```python
from build123d import *

# Parameters (mm, degrees)
F1_DEPTH    = 6
F2_T1_DEPTH = 28.6290423826
F3_W        = 12.6199351555
F3_H        = 2
F3_W_2      = 15.3329153147
F4_DEPTH    = 6


# Not quite as in the source:
# - a fillet or chamfer that OpenCascade refuses, or shapes differently, is made with other operations: its cross-section is extruded or revolved along the edge and cut away or added


with BuildPart() as f1:
    # F0 (on Top) → F1 (new body)
    with BuildSketch(Plane.XY):
        Polygon((0, 7), (-7, 5), (0, 5), align=None)
        Polygon((0, 5), (-7, 5), (-7, 0), (0, 0), (11, 0), (18, 0), (18, 5), (11, 5), align=None)
        Polygon((0, 0), (-7, 0), (0, -2), align=None)
        Polygon((11, 7), (11, 5), (18, 5), align=None)
        Polygon((18, 0), (11, 0), (11, -2), align=None)
    extrude(amount=F1_DEPTH)

    # F2: fillet of radius 6 on 4 edges, made by hand

    # F2_s2 → F2_t1 (cut)
    with BuildSketch(Plane.XY.offset(-11.3145211913)):
        with BuildLine():
            ThreePointArc((-2.6483267674, 6.2433352093), (-5.7900918887, 4.0873646023), (-7, 0.4741915235))
            Line((-7, 0.4741915235), (-7, 5))
            Line((-7, 5), (-2.6483267674, 6.2433352093))
        make_face()
        with BuildLine():
            ThreePointArc((-7, 4.5258084765), (-5.7900918887, 0.9126353977), (-2.6483267674, -1.2433352093))
            Line((-2.6483267674, -1.2433352093), (-7, 0))
            Line((-7, 0), (-7, 4.5258084765))
        make_face()
        with BuildLine():
            ThreePointArc((18, 0.4741915235), (16.7900918887, 4.0873646023), (13.6483267674, 6.2433352093))
            Line((13.6483267674, 6.2433352093), (18, 5))
            Line((18, 5), (18, 0.4741915235))
        make_face()
        with BuildLine():
            ThreePointArc((13.6483267674, -1.2433352093), (16.7900918887, 0.9126353977), (18, 4.5258084765))
            Line((18, 4.5258084765), (18, 0))
            Line((18, 0), (13.6483267674, -1.2433352093))
        make_face()
    extrude(amount=F2_T1_DEPTH, mode=Mode.SUBTRACT)

    # F3 (on face) → F4 (cut)
    with BuildSketch(Plane.XY.offset(6)):
        with Locations((-2.9576308128, 2.5)):
            Rectangle(F3_W, F3_H)
        with Locations((15.3141208924, 2.5)):
            Rectangle(F3_W_2, F3_H)
    extrude(amount=-F4_DEPTH, mode=Mode.SUBTRACT)


solid = f1.part
```
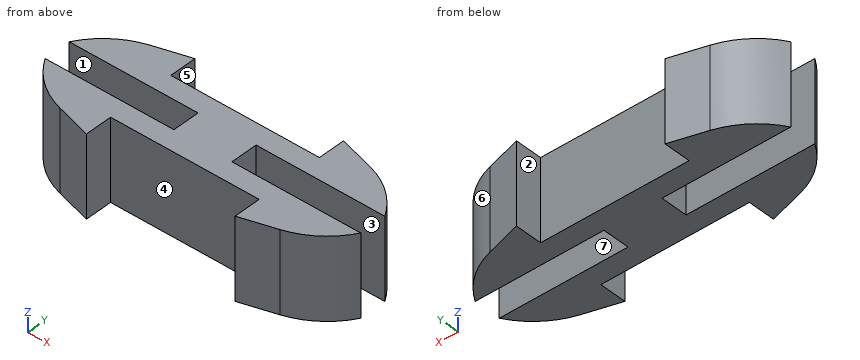
For this review, take the finished solid that the model builds, in its own axes (mm). Face numbers are marked on the shaded views. A direction names the side the tool comes from. Round coordinates to 2 decimals unless told otherwise and drop trailing zeros. Write each loop counter-clockwise with the first axis right and the second up, starting at its lowest first coordinate (ties: lowest second). Pieces come first, ordered by that corner, then holes. Notation, with made-up numbers: (89.25, 10.5) -> (105.25, 10.5) arc R15 cw to (105.25, 21.5) -> close; hole circle Ø3 at (-40, 56). An arc over 180 degrees is marked (long way). One line per question, with ' | ' between items. Start each with the question number.
(1) Mouldability with a two-part tool opening along X and no side actions: class the marked faces 4, 5, 6 and 7 as released by +X, released by -X, zero draft, split by the parting line, or undercut.
(2) Insertion check: P1, Ø1.6, axis at y = -1, z = 2.5, coming from the -X side; P2, Ø0.6, axis at y = 2.5, z = 3, coming from the -X side; P3, Ø2, axis at y = 6, z = 4.5, coming from the -X side. Each pin has a flat end and moves straight along its axis. Give the tip position at first contact, or say it passes through.
(3) Add section A-A, the plane x = 0.5. Write out the cut boundary in (y, z).
(4) Tool access review of the marked faces 1, 2 and 3: name each direction out of +Z, -Z, +X, -X, +Y, -Y from which nothing blocks a thin tool from reaching the whole face with its end or side.
(5) Add section C-C, the plane z = 3.25. Write out the cut boundary in (x, y), plus the area to 3 significant figures.
(6) Add section D-D, the plane y = 3.25. Write out the cut boundary in (x, z).
(7) For line 1 along Y through (x, z) = (3, 1.5); line 2 along Y through (x, z) = (-1.5, 2.5); line 3 along X through (y, z) = (2, 1), list the stretches that pass through material, from the lowest coordinate up. Write a range as from..to.
(8) Add section B-B, the plane y = 6.5. Write out the cut boundary in (x, z), plus the area to 3 significant figures.
Answer list:
1) face 4: undercut | face 5: undercut | face 6: released by +X | face 7: zero draft
2) P1: x = -4.7 | P2: x = 3.35 | P3: x = -4.94
3) outline: (0, 0) -> (1.5, 0) -> (1.5, 6) -> (0, 6) -> close; (3.5, 0) -> (5, 0) -> (5, 6) -> (3.5, 6) -> close
4) face 1: +Z, -Z, -X | face 2: +Z, -Z, +Y | face 3: +Z, -Z, +X
5) outline: (-6.18, 1.5) arc R6 ccw to (-2.65, -1.24) -> (0, -2) -> (0, 0) -> (11, 0) -> (11, -2) -> (13.65, -1.24) arc R6 ccw to (17.18, 1.5) -> (7.65, 1.5) -> (7.65, 3.5) -> (17.18, 3.5) arc R6 ccw to (13.65, 6.24) -> (11, 7) -> (11, 5) -> (0, 5) -> (0, 7) -> (-2.65, 6.24) arc R6 ccw to (-6.18, 3.5) -> (3.35, 3.5) -> (3.35, 1.5) -> close | area: 99.2 mm²
6) outline: (3.35, 0) -> (7.65, 0) -> (7.65, 6) -> (3.35, 6) -> close
7) line 1: 0..1.5, 3.5..5 | line 2: -1.57..1.5, 3.5..6.57 | line 3: 3.35..7.65
8) outline: (-1.75, 0) -> (0, 0) -> (0, 6) -> (-1.75, 6) -> close; (11, 0) -> (12.75, 0) -> (12.75, 6) -> (11, 6) -> close | area: 21.0 mm²
